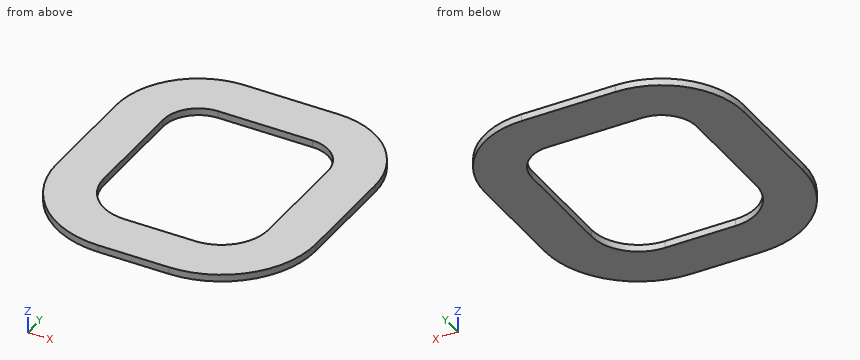
from build123d import *

# Parameters (mm, degrees)
BOSS_EXTRUDE1_DEPTH = 3


with BuildPart() as part:
    # Sketch1 → Boss-Extrude1 (new body)
    with BuildSketch(Plane.XY):
        with BuildLine():
            Line((-20, 52), (20, 52))
            ThreePointArc((20, 52), (44.748737342, 41.748737342), (55, 17))
            Line((55, 17), (55, -28))
            ThreePointArc((55, -28), (43.284271247, -56.284271247), (15, -68))
            Line((15, -68), (0.5, -68))
            Line((0.5, -68), (-0.5, -68))
            Line((-0.5, -68), (-15, -68))
            ThreePointArc((-15, -68), (-43.284271247, -56.284271247), (-55, -28))
            Line((-55, -28), (-55, 17))
            ThreePointArc((-55, 17), (-44.748737342, 41.748737342), (-20, 52))
        make_face()
        with BuildLine():
            Line((-20, 32), (20, 32))
            ThreePointArc((20, 32), (30.606601718, 27.606601718), (35, 17))
            Line((35, 17), (35, -28))
            ThreePointArc((35, -28), (29.142135624, -42.142135624), (15, -48))
            Line((15, -48), (0.5, -48))
            Line((0.5, -48), (-0.5, -48))
            Line((-0.5, -48), (-15, -48))
            ThreePointArc((-15, -48), (-29.142135624, -42.142135624), (-35, -28))
            Line((-35, -28), (-35, 17))
            ThreePointArc((-35, 17), (-30.606601718, 27.606601718), (-20, 32))
        make_face(mode=Mode.SUBTRACT)
    extrude(amount=BOSS_EXTRUDE1_DEPTH)


solid = part.part
Read the model definition and answer for the solid it produces. Units are mm, in the model's axes. Give positions to 0.01 mm unless a question says otherwise; leave off trailing zeros. Write each loop counter-clockwise with the first axis right and the second up, starting at its lowest first coordinate (ties: lowest second). Pieces come first, ordered by that corner, then holes. Notation, with made-up numbers: M 64,-26.5 L 93,-26.5 A13 ccw 93,-21.5 Z; hole C 71.5,32.25 d10. An arc over 180 degrees is marked long. One line per item, written item: value. Start each with the question number.
(1) Find the intervals of material crossed by line 1 (X direction, y = -8.5, z = 1.65); line 2 (Y direction, x = -2.5, z = 2.5); line 3 (X direction, y = -29.5, z = 1.8), in increasing order.
(2) Find section D-D (y = -60). Determine the outline of the cut face in (x, z).
(3) Find section B-B (x = 12.5). Determine the outline of the cut face in (y, z), plus the area to 3 significant figures.
(4) Find section C-C (z = 2.1). Determine the outline of the cut face in (x, y).
(5) Find section A-A (y = 12.5). Determine the outline of the cut face in (x, z).
Results below:
1. line 1: x = -55 to -35, 35 to 55
1. line 2: y = -68 to -48, 32 to 52
1. line 3: x = -54.97 to -34.94, 34.94 to 54.97
2. outline: M -39,0 L 39,0 L 39,3 L -39,3 Z
3. outline: M -68,0 L -48,0 L -48,3 L -68,3 Z; M 32,0 L 52,0 L 52,3 L 32,3 Z
3. area: 120 mm^2
4. outline: M -55,-28 A40 ccw -15,-68 L 15,-68 A40 ccw 55,-28 L 55,17 A35 ccw 20,52 L -20,52 A35 ccw -55,17 Z; hole M -35,-28 A20 ccw -15,-48 L 15,-48 A20 ccw 35,-28 L 35,17 A15 ccw 20,32 L -20,32 A15 ccw -35,17 Z
5. outline: M -55,0 L -35,0 L -35,3 L -55,3 Z; M 35,0 L 55,0 L 55,3 L 35,3 Z
